from build123d import *

# Parameters (mm, degrees)
F0_W     = 200
F0_H     = 100
F0_R     = 4
F0_R_2   = 11
F0_R_3   = 2
F1_DEPTH = 10
F0_R_4   = 7
F2_DEPTH = 3


with BuildPart() as f1:
    # F0 (on Top) → F1 (new body)
    with BuildSketch(Plane.XY):
        with Locations((-36.014734, 12.836266)):
            Rectangle(F0_W, F0_H)
        with Locations((-124.00907, -25.163734)):
            Circle(F0_R, mode=Mode.SUBTRACT)
        with Locations((-62.014734, -25.163734)):
            Circle(F0_R, mode=Mode.SUBTRACT)
        with Locations((-16.014734, -17.163734)):
            Circle(F0_R_2, mode=Mode.SUBTRACT)
        with Locations((-126.014734, 12.836266)):
            Circle(F0_R_3, mode=Mode.SUBTRACT)
        with Locations((-124.014734, 50.836266)):
            Circle(F0_R, mode=Mode.SUBTRACT)
        with Locations((-62.014734, 50.836266)):
            Circle(F0_R, mode=Mode.SUBTRACT)
        with Locations((-36.014734, 12.836266)):
            Circle(F0_R_3, mode=Mode.SUBTRACT)
        with Locations((53.985266, 12.836266)):
            Circle(F0_R_3, mode=Mode.SUBTRACT)
        with Locations((43.985266, 42.836266)):
            Circle(F0_R_2, mode=Mode.SUBTRACT)
    extrude(amount=F1_DEPTH)

    # F0 (on Top) → F2 (join)
    with BuildSketch(Plane.XY):
        with Locations((-16.014734, -17.163734)):
            Circle(F0_R_2)
        with Locations((-16.014734, -17.163734)):
            Circle(F0_R_4, mode=Mode.SUBTRACT)
        with Locations((43.985266, 42.836266)):
            Circle(F0_R_2)
        with Locations((43.985266, 42.836266)):
            Circle(F0_R_4, mode=Mode.SUBTRACT)
    extrude(amount=F2_DEPTH)


solid = f1.part
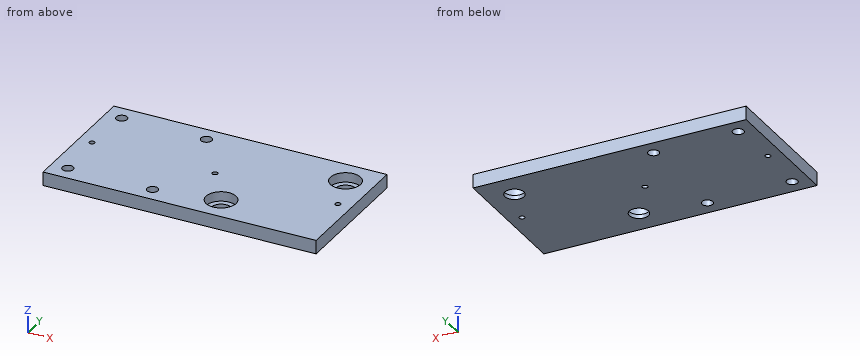
The model under review builds one solid part; all positions refer to its coordinate system, in mm. Round coordinates to 2 decimals unless told otherwise and drop trailing zeros. Loops run counter-clockwise (first coordinate to the right, second up) from the corner with the lowest first, then second, coordinate; pieces in that order, holes last. Notation, with made-up numbers: (31, 67.5) -> (61, 67.5) arc R21 ccw to (61, 89.5) -> close; hole circle Ø9 at (1.25, 3.25). An arc over 180 degrees is marked (long way). Write item = value, one per line. Start each with the question number.
Item 1: Take a section at B-B on x = -13.5. Give the boundary of the cut face in (y, z), plus the area to 3 significant figures.
Item 2: Insertion check: pin 1 (6.5 mm diameter, centred on x = 48.5, y = 42, fed in from +Z). The pin has a flat end and moves straight along its axis. Give the tip position at first contact, or say it passes through.
Item 3: Take a section at C-C on z = 1.5. Count the separate pieces of the cut face and the enclosed holes in it, plus the area to 3 significant figures.
Item 4: Take a section at A-A on y = -15. Give the boundary of the cut face in (x, z).
Item 5: To check wall thickness, follow L1, parallel to Y at x = -65, z = 5; L2, parallel to Y at x = -123, z = 6; L3, parallel to X at y = -16.5, z = 1.5. State the ranges of each line that lie inside material, in increasing order.
Result:
q1.outline = (-37.16, 0) -> (-23.7, 0) -> (-23.7, 3) -> (-27.87, 3) -> (-27.87, 10) -> (-37.16, 10) -> close; (-10.63, 0) -> (62.84, 0) -> (62.84, 10) -> (-6.46, 10) -> (-6.46, 3) -> (-10.63, 3) -> close
q1.area = 811 mm²
q2.pin_1 = 3
q3.separate_pieces = 1
q3.enclosed_holes = 9
q3.area = 19,500 mm²
q4.outline = (-136.01, 0) -> (-22.67, 0) -> (-22.67, 3) -> (-26.8, 3) -> (-26.8, 10) -> (-136.01, 10) -> close; (-9.36, 0) -> (63.99, 0) -> (63.99, 10) -> (-5.23, 10) -> (-5.23, 3) -> (-9.36, 3) -> close
q5.L1 = -37.16 to -27.83, -22.5 to 48.17, 53.5 to 62.84
q5.L2 = -37.16 to -29.03, -21.29 to 46.97, 54.71 to 62.84
q5.L3 = -136.01 to -22.98, -9.05 to 63.99
